The listing builds one solid part. Answer for the finished solid, in the listing's coordinates (mm). Face numbers are marked on the shaded views. A direction names the side the tool comes from. Round coordinates to 2 decimals unless told otherwise and drop trailing zeros. Loops run counter-clockwise (first coordinate to the right, second up) from the corner with the lowest first, then second, coordinate; pieces in that order, holes last. Notation, with made-up numbers: M 24.25,21 L 34.25,21 A20 cw 34.25,56 Z; hole C 64.5,-19.5 d4. An arc over 180 degrees is marked long. Put each result on its own line as item: value. Start each with the question number.
(1) Section A-A, the plane x = 0 is taken. Determine the outline of the cut face in (y, z), then the cut area to 3 significant figures.
(2) Straight lines are drawn through the part: line 1 (X direction, y = 33.25, z = 0); line 2 (X direction, y = 34.55, z = 0); line 3 (X direction, y = 21, z = 0). For each, find the intervals that lie inside material, in ascending order.
(3) Section D-D, the plane y = 12 is taken. Determine the outline of the cut face in (x, z).
(4) Section B-B, the plane z = 0 is taken. Count the separate pieces of the cut face and the enclosed holes in it, then the cut area to 3 significant figures.
(5) Section C-C, the plane z = -14 is taken. Determine the outline of the cut face in (x, y), then the cut area to 3 significant figures.
(6) Which of the six approach directions +Z, -Z, +X, -X, +Y, -Y give full straight-line access (tool end or side, diameter ignored) to the marked faces 4, 5, 6, 7 and 8?
(7) Flat-ended cylindrical pins translate along their axes: P1, Ø14, axis at x = -2.5, z = -7.5, coming from the -Y side; P2, Ø6, axis at y = 8, z = -11, coming from the +X side; P3, Ø7.5, axis at x = -33.5, y = 35.5, coming from the -Z side; P4, Ø5.5, axis at x = 30, y = 35, coming from the +Z side. Find the tip coordinate at first contact, or state that the pin passes through.
(8) Determine the mould class of the marked faces 1, 2 and 3 for opening direction X: released by +X, released by -X, zero draft, split by the parting line, or undercut.
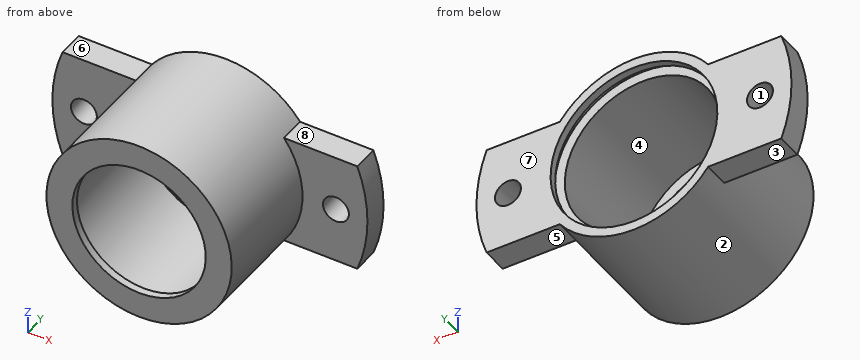
```python
from build123d import *

# Parameters (mm, degrees)
BOSS_EXTRUDE2_START = -7
BOSS_EXTRUDE2_DEPTH = 7
SKETCH8_R           = 3.5
CUT_EXTRUDE2_DEPTH  = 7


with BuildPart() as part:
    # Sketch4 → Revolve1 (revolve)
    with BuildSketch(Plane(origin=(0, 0, 0), x_dir=(0, 0, -1), z_dir=(1, 0, 0)), mode=Mode.PRIVATE) as revolve1_sk:
        Polygon((-25, 37.75), (-25, 0), (-18, 0), (-18, 2), (-21, 2), (-21, 34), (-23.75, 34), (-23.75, 35.75), (-22.5, 35.75), (-22.5, 37.75), align=None)
    revolve(revolve1_sk.sketch.rotate(Axis((0, -1.117924861, 0), (0, 1, 0)), 180), axis=Axis((0, -1.117924861, 0), (0, 1, 0)))

    # Sketch7 → Boss-Extrude2 (add)
    with BuildSketch(Plane(origin=(0, 37.75, 0), x_dir=(1, 0, 0), z_dir=(0, 1, 0)).offset(BOSS_EXTRUDE2_START)):
        with BuildLine():
            Line((-39.764934301, -15), (-20, -15))
            ThreePointArc((-20, -15), (-25, 0), (-20, 15))
            Line((-20, 15), (-39.764934301, 15))
            ThreePointArc((-39.764934301, 15), (-42.5, 0), (-39.764934301, -15))
        make_face()
        with BuildLine():
            Line((39.764934301, 15), (20, 15))
            ThreePointArc((20, 15), (25, 0), (20, -15))
            Line((20, -15), (39.764934301, -15))
            ThreePointArc((39.764934301, -15), (42.5, 0), (39.764934301, 15))
        make_face()
    extrude(amount=BOSS_EXTRUDE2_DEPTH)

    # Sketch8 → Cut-Extrude2 (cut)
    with BuildSketch(Plane(origin=(0, 37.75, 0), x_dir=(1, 0, 0), z_dir=(0, 1, 0))):
        with Locations(Location((34, 0, 0), (0, 0, 270))):
            Circle(SKETCH8_R)
        with Locations(Location((-34, 0, 0), (0, 0, 270))):
            Circle(SKETCH8_R)
    extrude(amount=-CUT_EXTRUDE2_DEPTH, mode=Mode.SUBTRACT)


solid = part.part
```
Recorded:
1. outline: M 0,-25 L 37.75,-25 L 37.75,-22.5 L 35.75,-22.5 L 35.75,-23.75 L 34,-23.75 L 34,-21 L 2,-21 L 2,-18 L 0,-18 Z; M 0,18 L 2,18 L 2,21 L 34,21 L 34,23.75 L 35.75,23.75 L 35.75,22.5 L 37.75,22.5 L 37.75,25 L 0,25 Z
1. area: 298 mm²
2. line 1: x = -42.5 to -37.5, -30.5 to -21, 21 to 30.5, 37.5 to 42.5
2. line 2: x = -42.5 to -37.5, -30.5 to -23.75, 23.75 to 30.5, 37.5 to 42.5
2. line 3: x = -25 to -21, 21 to 25
3. outline: C 0,0 d50; hole C 0,0 d42
4. separate pieces: 4
4. enclosed holes: 0
4. area: 445 mm²
5. outline: M -40.13,30.75 L -20.71,30.75 L -20.71,0 L -11.31,0 L -11.31,2 L -15.65,2 L -15.65,34 L -19.18,34 L -19.18,35.75 L -17.61,35.75 L -17.61,37.75 L -40.13,37.75 Z; M 11.31,0 L 20.71,0 L 20.71,30.75 L 40.13,30.75 L 40.13,37.75 L 17.61,37.75 L 17.61,35.75 L 19.18,35.75 L 19.18,34 L 15.65,34 L 15.65,2 L 11.31,2 Z
5. area: 651 mm²
6. face 4: +Y
6. face 5: -Z, +X, +Y, -Y
6. face 6: +Z, -X, +Y, -Y
6. face 7: +Z, -Z, +X, -X, +Y
6. face 8: +Z, +X, +Y, -Y
7. P1: passes through
7. P2: stops at x = 23.69
7. P3: stops at z = -15
7. P4: stops at z = 15
8. face 1: undercut
8. face 2: split by the parting line
8. face 3: zero draft
